The listing builds one solid part. Answer for the finished solid, in the listing's coordinates (mm). Give positions to 0.01 mm unless a question says otherwise; leave off trailing zeros. Loops run counter-clockwise (first coordinate to the right, second up) from the corner with the lowest first, then second, coordinate; pieces in that order, holes last. Notation, with made-up numbers: (46.25, 55) - (90.25, 55) arc R15 cw to (90.25, 73) - close; hole circle Ø8 at (-32, -5). An arc over 180 degrees is marked (long way). Answer as CSV lines item,"result". Start each with the question number.
1) Find the intervals of material crossed by line 1 along Y through (x, z) = (-473, 1); line 2 along X through (y, z) = (106, -7); line 3 along Z through (x, y) = (-922.85, 690), in increasing order.
2) A cutting plane is placed at B-B (x = 572). Determine the outline of the cut face in (y, z).
3) A cutting plane is placed at C-C (y = -580). Determine the outline of the cut face in (x, z), and give its area (3 significant figures).
Autodesk Inventor part; units mm, degrees
ref_plane "YZ Plane" through (0, 0, 0) normal (1, 0, 0) x (0, 1, 0)
ref_plane "XZ Plane" through (0, 0, 0) normal (0, 1, 0) x (-1, 0, 0)
ref_plane "XY Plane" through (0, 0, 0) normal (0, 0, 1) x (1, 0, 0)
sketch "Sketch1" plane through (0, 0, 0) normal (0, 0, 1) x (1, 0, 0)
  line L0 (920, -1050) -> (-920, -1050)
  line L1 (-920, -1050) -> (-920, 1050)
  line L2 (-920, 1050) -> (920, 1050)
  line L3 (920, 1050) -> (920, -1050)
  line L4 (920, -1050) -> (-920, 1050) construction
  line L5 (-920, -1050) -> (920, 1050) construction
  line L6 (924, 1054) -> (-924, 1054)
  line L7 (-924, 1054) -> (-924, -1054)
  line L8 (-924, -1054) -> (924, -1054)
  line L9 (924, -1054) -> (924, 1054)
  point P0 (0, 0)
  dimension "d0" = 1840
  dimension "d1" = 2100
  dimension "d2" = 4
extrude "Extrusion1" add sketch "Sketch1" along normal mid plane 40
sketch "Sketch2" plane through (-920, -1050, 20) normal (1, 0, 0) x (0, 0, -1)
  line L0 (0, 2104) -> (0, -4)
  line L1 (40, -4) -> (40, 2104)
  line L2 (0, 1750) -> (40, 1750)
  line L3 (40, 1750) -> (40, 1650)
  line L4 (40, 1650) -> (0, 1650)
  line L5 (0, 1650) -> (0, 1750)
  line L6 (0, 2104) -> (40, 2104)
  line L7 (0, 1050) -> (40, 1050)
  line L8 (40, 1050) -> (40, 950)
  line L9 (0, 950) -> (0, 1050)
  line L10 (40, 950) -> (0, 950)
  line L11 (0, 350) -> (40, 350)
  line L12 (40, 350) -> (40, 250)
  line L13 (0, 250) -> (0, 350)
  line L14 (40, 250) -> (0, 250)
  line L15 (40, 2100) -> (0, 2100)
  point P0 (20, 1050)
  point P1 (0, 250)
  point P2 (40, 350)
  point P3 (0, 950)
  point P4 (40, 1050)
  point P5 (0, 1650)
  point P6 (40, 1750)
  dimension "d5" = 100
  dimension "d9" = 700
  dimension "d24" = 350
extrude "Extrusion2" cut sketch "Sketch2" against normal blind 2.5 contours L2 L1 L4 L0 | L7 L1 L10 L0 | L11 L1 L14 L0
mirror "Mirror1" about plane through (0, 0, 0) normal (1, 0, 0) of "Extrusion2"
sketch "Sketch3" plane through (-922.5, -1050, 20) normal (1, 0, 0) x (0, 0, -1)
  circle A0 centre (20, 340) radius 4
  line L0 (0, 2104) -> (0, -4)
  line L1 (0, 350) -> (40, 350)
  point P0 (20, 1050)
  dimension "d16" = 8
  dimension "d17" = 20
  dimension "d18" = 10
extrude "Extrusion3" cut sketch "Sketch3" against normal blind 1
pattern_linear "Rectangular Pattern1" count 3 spacing 700 along (0, 1, 0) of "Extrusion3"
mirror "Mirror2" about plane through (0, 0, 0) normal (1, 0, 0) of "Extrusion3", "Rectangular Pattern1"
properties part number "Frame2" material "Zinc"
Ans:
1,line 1,"-1054 to -1050, 1050 to 1054"
1,line 2,"-924 to -920, 920 to 924"
1,line 3,"-20 to -4, 4 to 20"
2,outline,"(-1054, -20) - (-1050, -20) - (-1050, 20) - (-1054, 20) - close; (1050, -20) - (1054, -20) - (1054, 20) - (1050, 20) - close"
3,outline,"(-924, -20) - (-920, -20) - (-920, 20) - (-924, 20) - close; (920, -20) - (924, -20) - (924, 20) - (920, 20) - close"
3,area,"320 mm2"
